```python
from build123d import *

# Parameters (mm, degrees)
SKETCH_1_R               = 3
EXTRUDE_1_DEPTH          = 11
SKETCH_2_R               = 1.5
CUT_EXTRUDE_1_DEPTH      = 5
CUT_EXTRUDE_2_DEPTH      = 12.789826123
CUT_EXTRUDE_2_DEPTH_BACK = 12.789826123
SKETCH_3_R               = 1.5
SKETCH_3_R_2             = 0.5
CUT_EXTRUDE_3_DEPTH      = 12.789826267
CUT_EXTRUDE_3_DEPTH_BACK = 12.789826267
SKETCH_4_W               = 2.5
SKETCH_4_H               = 5
EXTRUDE_START            = 2
SKETCH_5_R               = 3
SKETCH_5_R_2             = 1.5
EXTRUDE_2_DEPTH          = 2


with BuildPart() as part:
    # 草图1 → 凸台-拉伸1 (new body)
    with BuildSketch(Plane(origin=(0, 0, 0), x_dir=(1, 0, 0), z_dir=(0, 1, 0))):
        with Locations(Location((0, 0, 0), (0, 0, 270))):
            Circle(SKETCH_1_R)
    extrude(amount=EXTRUDE_1_DEPTH)

    # 草图2 → 切除-拉伸1 (cut)
    with BuildSketch(Plane.XZ):
        with Locations(Location((0, 0, 0), (0, 0, 270))):
            Circle(SKETCH_2_R)
    extrude(amount=-CUT_EXTRUDE_1_DEPTH, mode=Mode.SUBTRACT)

    # 草图3 → 切除-拉伸2 (cut, two sides: drawn at the far end of the back side and taken through both)
    with BuildSketch(Plane(origin=(0, 0, 0), x_dir=(0, 0, -1), z_dir=(1, 0, 0)).offset(-CUT_EXTRUDE_2_DEPTH_BACK)):
        with Locations((0, 8.5)):
            Circle(SKETCH_3_R)
        with Locations((0, 2.5)):
            Circle(SKETCH_3_R_2)
        with BuildLine():
            Line((-3, 8.5), (-3, 11))
            Line((-3, 11), (-1.658168408, 11.000095504))
            ThreePointArc((-1.658168408, 11.000095504), (-2.643341183, 9.918713286), (-3, 8.5))
        make_face()
        with BuildLine():
            Line((1.658168408, 11.000095504), (3, 11))
            Line((3, 11), (3, 8.5))
            ThreePointArc((3, 8.5), (2.643341183, 9.918713286), (1.658168408, 11.000095504))
        make_face()
    extrude(amount=CUT_EXTRUDE_2_DEPTH + CUT_EXTRUDE_2_DEPTH_BACK, mode=Mode.SUBTRACT)

    # 草图4 → 切除-拉伸3 (cut, two sides: drawn at the far end of the back side and taken through both)
    with BuildSketch(Plane.XY.offset(-CUT_EXTRUDE_3_DEPTH_BACK)):
        with Locations((0, 8.5)):
            Rectangle(SKETCH_4_W, SKETCH_4_H)
    extrude(amount=CUT_EXTRUDE_3_DEPTH + CUT_EXTRUDE_3_DEPTH_BACK, mode=Mode.SUBTRACT)

    # 草图5 → 凸台-拉伸2 (add)
    with BuildSketch(Plane.XZ.offset(EXTRUDE_START)):
        with Locations(Location((0, 0, 0), (0, 0, 270))):
            Circle(SKETCH_5_R)
        with Locations(Location((0, 0, 0), (0, 0, 270))):
            Circle(SKETCH_5_R_2, mode=Mode.SUBTRACT)
    extrude(amount=-EXTRUDE_2_DEPTH)


solid = part.part
```
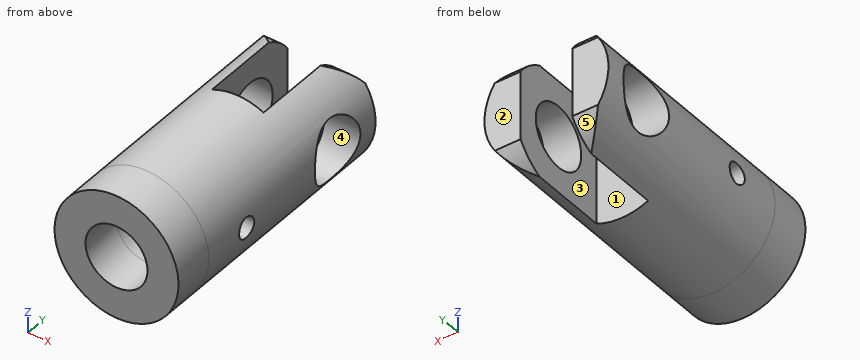
Geometry: final body of the model. Coordinates: model frame, mm. Face numbers are marked on the shaded views. A direction names the side the tool comes from. Give positions to 0.01 mm unless a question says otherwise; leave off trailing zeros. Write each loop counter-clockwise with the first axis right and the second up, starting at its lowest first coordinate (ties: lowest second). Pieces come first, ordered by that corner, then holes.
1. Reachability of the marked faces 1 and 2 from +Z, -Z, +X, -X, +Y, -Y: full face, straight path, thin tool, end or side. Return the list, or none.
2. Line query: probe 1 along Y at (x, z) = (2.3, 0); probe 2 along X at (y, z) = (-0.25, 0); probe 3 along Y at (x, z) = (-2.5, 0.25). Output: solid intervals per line, ascending.
3. Section query A-A, the plane z = 0. Return loops of the section in (x, y), then the cut area to 3 significant figures.
4. Section query C-C, the plane y = 2.5. Return loops of the section in (x, z).
5. Section query D-D, the plane x = 0.75. Return loops of the section in (y, z), then the cut area to 3 significant figures.
6. Section query B-B, the plane y = 8. Return loops of the section in (x, z).
7. Draft query along Y for the marked faces 3, 4 and 5. Return one class per face: released by +Y, released by -Y, zero draft, split by the parting line, or undercut.
8. Pin query (flat end, axial travel): P1, Ø2.5, axis at x = 0.5, z = -0.5, coming from the -Y side; P2, Ø3, axis at x = -1.5, y = 7, coming from the -Z side; P3, Ø1.3, axis at x = -0.5, z = -0.5, coming from the +Y side; P4, Ø2.5, axis at y = 8.5, z = 0, coming from the -X side. Return the tip coordinate at first contact, or that it passes through.
Computed:
1. face 1: +Z, -Z, +Y
1. face 2: +Z, -Z, +X, -X, +Y
2. probe 1: y = -2 to 2, 3 to 7, 10 to 11
2. probe 2: x = -3 to -1.5, 1.5 to 3
2. probe 3: y = -2 to 2.07, 2.93 to 7.02, 9.98 to 11
3. outline: (-3, -2) - (-1.5, -2) - (-1.5, 2) - (-3, 2) - close; (-3, 3) - (-1.5, 3) - (-1.5, 5) - (1.5, 5) - (1.5, 3) - (3, 3) - (3, 7) - (1.25, 7) - (1.25, 6) - (-1.25, 6) - (-1.25, 7) - (-3, 7) - close; (-3, 10) - (-1.25, 10) - (-1.25, 11) - (-3, 11) - close; (1.25, 10) - (3, 10) - (3, 11) - (1.25, 11) - close; (1.5, -2) - (3, -2) - (3, 2) - (1.5, 2) - close
3. area: 31.0 mm2
4. outline: (-2.96, -0.5) arc R3 ccw to (2.96, -0.5) - (1.41, -0.5) arc R1.5 cw to (-1.41, -0.5) - close; (-2.96, 0.5) - (-1.41, 0.5) arc R1.5 cw to (1.41, 0.5) - (2.96, 0.5) arc R3 ccw to start
5. outline: (-2, -2.9) - (6, -2.9) - (6, 2.9) - (-2, 2.9) - (-2, 1.3) - (5, 1.3) - (5, -1.3) - (-2, -1.3) - close
5. area: 28.3 mm2
6. outline: (-2.65, -1.41) arc R3 ccw to (-1.25, -2.73) - (-1.25, -1.41) - close; (-2.65, 1.41) - (-1.25, 1.41) - (-1.25, 2.73) arc R3 ccw to start; (1.25, -2.73) arc R3 ccw to (2.65, -1.41) - (1.25, -1.41) - close; (1.25, 1.41) - (2.65, 1.41) arc R3 ccw to (1.25, 2.73) - close
7. face 3: zero draft
7. face 4: undercut
7. face 5: released by +Y
8. P1: stops at y = -2
8. P2: stops at z = -2.98
8. P3: stops at y = 6
8. P4: passes through
